Here's how the part is built. I have some questions about the finished solid (model axes, mm). Face numbers are marked on the shaded views. A direction names the side the tool comes from. Give positions to 0.01 mm unless a question says otherwise; leave off trailing zeros. Loops run counter-clockwise (first coordinate to the right, second up) from the corner with the lowest first, then second, coordinate; pieces in that order, holes last. Notation, with made-up numbers: (33, 15) - (70, 15) arc R24 cw to (70, 29) - close; hole circle Ø6 at (-5, 76.5). An arc over 180 degrees is marked (long way). One line per item, written item: value. Start each with the question number.
Solid Edge part; units mm, degrees
sketch "Sketch1" plane through (0, 0, 0) normal (0, -1, 0) x (1, 0, 0)
  line L0 (-47.5, -18.75) -> (47.5, -18.75)
  line L1 (47.5, -18.75) -> (47.5, 18.75)
  line L2 (47.5, 18.75) -> (-47.5, 18.75)
  line L3 (-47.5, 18.75) -> (-47.5, -18.75)
extrude "Ajout_matière_1" add sketch "Sketch1" along normal blind 2
hole "Perçage_1" at (-43.5, 0, 16.75) direction (0, -1, 0) diameter 2 end through all
hole "Hole1" at (42.5, 0, -13.25) direction (0, -1, 0) diameter 2 end through all
hole "Hole2" at (23.5, 0, -9.75) direction (0, -1, 0) diameter 2 end through all
hole "Hole3" at (39.5, 0, 16.75) direction (0, -1, 0) diameter 2 end through all
sketch "Sketch2" plane through (0, 0, 0) normal (0, 1, 0) x (1, 0, 0)
  line L0 (-47.5, 18.75) -> (47.5, 18.75)
  line L1 (47.5, 18.75) -> (47.5, -18.75)
  line L2 (47.5, -18.75) -> (-47.5, -18.75)
  line L3 (-47.5, -18.75) -> (-47.5, 18.75)
  line L4 (-49.5, -20.75) -> (49.5, -20.75)
  line L5 (49.5, -20.75) -> (49.5, 20.75)
  line L6 (49.5, 20.75) -> (-49.5, 20.75)
  line L7 (-49.5, 20.75) -> (-49.5, -20.75)
  dimension "D1" = 49.5
  dimension "D2" = 49.5
extrude "Ajout_matière_2" add sketch "Sketch2" against normal blind 2
sketch "Sketch3" plane through (0, 0, 0) normal (0, 1, 0) x (1, 0, 0)
  line L0 (-32.5, -11.75) -> (-22.5, -11.75)
  line L1 (-22.5, -11.75) -> (-22.5, 13.25)
  line L2 (-22.5, 13.25) -> (-32.5, 13.25)
  line L3 (-32.5, 13.25) -> (-32.5, -11.75)
  dimension "D1" = 32.5
  dimension "D2" = 22.5
  dimension "D3" = 32.5
extrude "Ajout_matière_3" add sketch "Sketch3" along normal blind 8
sketch "Sketch4" plane through (0, 0, 0) normal (0, 1, 0) x (1, 0, 0)
  line L0 (-21.5, -11.75) -> (-11.5, -11.75)
  line L1 (-11.5, -11.75) -> (-11.5, 11.25)
  line L2 (-11.5, 11.25) -> (-21.5, 11.25)
  line L3 (-21.5, 11.25) -> (-21.5, -11.75)
  dimension "D1" = 21.5
  dimension "D2" = 11.5
  dimension "D3" = 11.5
extrude "Ajout_matière_4" add sketch "Sketch4" along normal blind 4
sketch "Sketch5" plane through (0, 0, 0) normal (0, 1, 0) x (1, 0, 0)
  line L0 (-4.5, -6.25) -> (35.5, -6.25)
  line L1 (35.5, -6.25) -> (35.5, 6.75)
  line L2 (35.5, 6.75) -> (-4.5, 6.75)
  line L3 (-4.5, 6.75) -> (-4.5, -6.25)
  dimension "D1" = 35.5
  dimension "D2" = 35.5
extrude "Ajout_matière_5" add sketch "Sketch5" along normal blind 7
sketch "Sketch6" plane through (0, 0, 0) normal (0, 1, 0) x (1, 0, 0)
  line L0 (41.5, -5.25) -> (59.5, -5.25)
  line L1 (59.5, -5.25) -> (59.5, 5.75)
  line L2 (59.5, 5.75) -> (41.5, 5.75)
  line L3 (41.5, 5.75) -> (41.5, -5.25)
  dimension "D1" = 59.5
  dimension "D2" = 59.5
extrude "Ajout_matière_6" add sketch "Sketch6" along normal blind 6
sketch "Sketch7" plane through (0, 0, 0) normal (0, 1, 0) x (0, 0, -1)
  line L0 (-11.75, 46.5) -> (0.25, 46.5)
  line L1 (0.25, 46.5) -> (0.25, 41.5)
  line L2 (0.25, 41.5) -> (-11.75, 41.5)
  line L3 (-11.75, 41.5) -> (-11.75, 46.5)
  dimension "D1" = 11.75
  dimension "D2" = 0.25
  dimension "D3" = 11.75
extrude "Ajout_matière_7" add sketch "Sketch7" along normal blind 3.5
sketch "Sketch8" plane through (0, 0, 0) normal (0, 1, 0) x (0, 0, -1)
  circle A0 centre (-9.25, 6) radius 2.5
  circle A1 centre (-9.25, -2) radius 2.5
  circle A2 centre (-9.25, -10) radius 2.5
  circle A3 centre (11.75, 36) radius 2.5
  dimension "D1" = 9.25
extrude "Ajout_matière_8" add sketch "Sketch8" along normal blind 6
properties material "Epoxy, rigide"
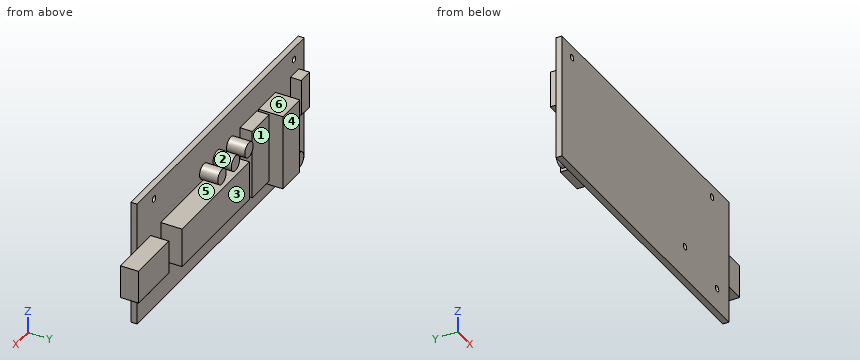
(1) If we section it at B-B on x = 15: List the corners of the cut face in (y, z) for me, plus the area to 3 significant figures.
(2) If we section it at D-D on x = -12.5: List the corners of the cut face in (y, z) for me.
(3) Will these pins go through, and if not, where does the flat tip stop? pin 1 (1.8 mm diameter, centred on x = 52, y = 2.5, fed in from +Z); pin 2 (4.5 mm diameter, centred on y = 3, z = 6, fed in from -X); pin 3 (3 mm diameter, centred on y = 5, z = 8, fed in from +X); pin 4 (1.2 mm diameter, centred on x = 39.5, z = 16.75, fed in from -Y).
(4) If we section it at C-C on z = -4.5: List the corners of the cut face in (x, y) for me, plus the area to 3 significant figures.
(5) If we mould it in two halves opening along Z, with no side actions, what happens to the marked faces 4, 5 and 6? For each: pulls with the +Z half, pulls with the -Z half, needs draft (parallel to the pull), parting line crosses it, or undercut.
(6) Please list where these lines run through material, in increasing order: probe 1 along X at (y, z) = (-0.55, 16.75); probe 2 along Z at (x, y) = (39.5, -1.4); probe 3 along X at (y, z) = (-1.05, -9.75). Write a range as from..to.
(7) For the marked faces 1, 2 and 3, which set-ups out of +Z, -Z, +X, -X, +Y, -Y let a thin tool reach every point of the face, with its end or its side?
(8) If we section it at A-A on x = 42.5: List the corners of the cut face in (y, z) for me.
Found:
1. outline: (-2, -20.75) - (0, -20.75) - (0, -6.75) - (7, -6.75) - (7, 6.25) - (0, 6.25) - (0, 20.75) - (-2, 20.75) - close
1. area: 174 mm^2
2. outline: (-2, -20.75) - (0, -20.75) - (0, -11.25) - (4, -11.25) - (4, 11.75) - (0, 11.75) - (0, 20.75) - (-2, 20.75) - close
3. pin 1: z = 5.25
3. pin 2: x = -46.5
3. pin 3: x = 12.5
3. pin 4: through
4. outline: (-49.5, -2) - (49.5, -2) - (49.5, 0) - (59.5, 0) - (59.5, 6) - (41.5, 6) - (41.5, 0) - (35.5, 0) - (35.5, 7) - (-4.5, 7) - (-4.5, 0) - (-11.5, 0) - (-11.5, 4) - (-21.5, 4) - (-21.5, 0) - (-22.5, 0) - (-22.5, 8) - (-32.5, 8) - (-32.5, 0) - (-49.5, 0) - close
4. area: 706 mm^2
5. face 4: needs draft
5. face 5: undercut
5. face 6: pulls with the +Z half
6. probe 1: -49.5..-44.5, -42.5..38.5, 40.5..49.5
6. probe 2: -20.75..15.75, 17.75..20.75
6. probe 3: -49.5..22.5, 24.5..49.5
7. face 1: +Z, -Z, +Y
7. face 2: +Y
7. face 3: +Z, -Z, +X, +Y
8. outline: (-2, -20.75) - (0, -20.75) - (0, -14.25) - (-2, -14.25) - close; (-2, -12.25) - (0, -12.25) - (0, -5.75) - (6, -5.75) - (6, 5.25) - (0, 5.25) - (0, 20.75) - (-2, 20.75) - close
